from build123d import *

# Parameters (mm, degrees)
SKETCH2_W           = 290
SKETCH2_H           = 165.1
BOSS_EXTRUDE1_DEPTH = 51
SKETCH3_W           = 290
SKETCH3_H           = 165.1
BOSS_EXTRUDE2_DEPTH = 3.175
CUT_EXTRUDE1_DEPTH  = 161.925
SKETCH7_W           = 7.175
SKETCH7_H           = 41.725
CUT_EXTRUDE3_DEPTH  = 158.75
FILLET1_R           = 3.175
SKETCH8_W           = 290
SKETCH8_H           = 6.1
CUT_EXTRUDE4_DEPTH  = 3.25


with BuildPart() as part:
    # Sketch2 → Boss-Extrude1 (new body)
    with BuildSketch(Plane.XY):
        Rectangle(SKETCH2_W, SKETCH2_H)
        Polygon((133.825, 71.375), (133.825, -71.375), (133.825, -79.375), (-133.825, -79.375), (-133.825, -71.375), (-133.825, 71.375), (-133.825, 79.375), (133.825, 79.375), align=None, mode=Mode.SUBTRACT)
    extrude(amount=BOSS_EXTRUDE1_DEPTH)

    # Sketch3 → Boss-Extrude2 (add)
    with BuildSketch(Plane.XY.offset(51)):
        Rectangle(SKETCH3_W, SKETCH3_H)
    extrude(amount=BOSS_EXTRUDE2_DEPTH)

    # Sketch4 → Cut-Extrude1 (cut)
    with BuildSketch(Plane.XZ.offset(82.55)):
        Polygon((140.9, 2.9), (136.9, 2.9), (136.9, 6.1), (145, 6.1), (145, 2.9), (145, 0), (140.9, 0), align=None)
    cut_extrude1 = extrude(amount=-CUT_EXTRUDE1_DEPTH, mode=Mode.SUBTRACT)

    # Mirror1: Cut-Extrude1 across plane
    add(cut_extrude1.mirror(Plane(origin=(0, 0, 0), x_dir=(0, 0, 1), z_dir=(1, 0, 0))), mode=Mode.SUBTRACT)

    # Sketch7 → Cut-Extrude3 (cut)
    with BuildSketch(Plane(origin=(0, 79.375, 0), x_dir=(1, 0, 0), z_dir=(0, 1, 0))):
        with Locations((137.4125, -30.1375)):
            Rectangle(SKETCH7_W, SKETCH7_H)
    cut_extrude3 = extrude(amount=-CUT_EXTRUDE3_DEPTH, mode=Mode.SUBTRACT)

    # Mirror4: Cut-Extrude3 across plane
    add(cut_extrude3.mirror(Plane(origin=(0, 0, 0), x_dir=(0, 0, 1), z_dir=(1, 0, 0))), mode=Mode.SUBTRACT)

    # Fillet1
    fillet1_edges = [part.edges().sort_by_distance(p)[0] for p in [
        (145, -82.55, 30.1375),
        (-145, -82.55, 30.1375),
        (-145, 82.55, 27.0875),
        (145, 82.55, 27.0875),
    ]]
    fillet(fillet1_edges, radius=FILLET1_R)

    # Sketch8 → Cut-Extrude4 (cut)
    with BuildSketch(Plane.XZ.offset(82.55)):
        with Locations((0, 3.05)):
            Rectangle(SKETCH8_W, SKETCH8_H)
    extrude(amount=-CUT_EXTRUDE4_DEPTH, mode=Mode.SUBTRACT)


solid = part.part
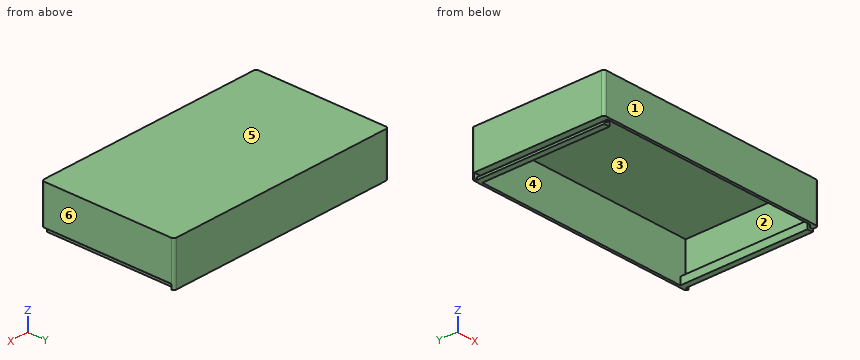
Part model, mm, in its own coordinate system. Face numbers are marked on the shaded views. A direction names the side the tool comes from. Coordinates: 2 decimals unless noted, no trailing zeros. Loops run counter-clockwise (first coordinate to the right, second up) from the corner with the lowest first, then second, coordinate; pieces in that order, holes last. Notation, with made-up numbers: M -23.75,-40 L 34.25,-40 A23 ccw 34.25,-4 Z; hole C -26,59.5 d1. An arc over 180 degrees is marked long. Use a Markdown table: item, result. Add a question column.
Q1. Cut at B-B (z = 13). Write the cut outline in (x, y) (3 decimals).
Q2. Which spindle directions (+Z, -Z, +X, -X, +Y, -Y) get a long thin tool onto all of the face, cutting with end or side? Do the marked faces 1 and 2. Say none if no direction does.
Q3. Probe L1, parallel to X at y = -43.5, z = 16; L2, parallel to Y at x = -6, z = 34 (3 decimals); L3, parallel to X at y = 46, z = 5 (3 decimals). List the from-to ranges inside material, lowest first.
Q4. Cut at C-C (y = 66). Write the cut outline in (x, z) (3 decimals), and give its area (3 significant figures).
Q5. Cut at A-A (x = -12). Write the cut outline in (y, z) (3 decimals).
Q6. Pin check, flat tips, straight feed: P1, Ø2, axis at x = -37, y = 5.5, coming from the -Z side; P2, Ø1.4, axis at y = 29, z = 1, coming from the +X side; P3, Ø5, axis at x = 135.5, z = 2.5, coming from the -Y side; P4, Ø5, axis at x = -139, z = 4.5, coming from the -Y side. Stop position of each tip, or through.
Q7. Mould opens along X. For the marked faces 3, 4, 5 and 6 say: +X half, -X half, draft (parallel to the pull), parting line (faces both ways), or undercut.
Worked out:
| question | item | result |
|---|---|---|
| 1 | outline | M -145,-79.375 A3.175 ccw -141.825,-82.55 L 141.825,-82.55 A3.175 ccw 145,-79.375 L 145,79.375 A3.175 ccw 141.825,82.55 L -141.825,82.55 A3.175 ccw -145,79.375 Z; hole M -141,-79.375 L 141,-79.375 L 141,79.375 L -141,79.375 Z |
| 2 | face 1 | +Z, -Z, +X, -X, -Y |
| 2 | face 2 | none |
| 3 | L1 | x = -145 to -141, 141 to 145 |
| 3 | L2 | y = -82.55 to -79.375, 79.375 to 82.55 |
| 3 | L3 | x = -136.9 to -133.825, 133.825 to 136.9 |
| 4 | outline | M -145,6.1 L -136.9,6.1 L -136.9,2.9 L -140.9,2.9 L -140.9,0 L -133.825,0 L -133.825,9.275 L -141,9.275 L -141,51 L 141,51 L 141,9.275 L 133.825,9.275 L 133.825,0 L 140.9,0 L 140.9,2.9 L 136.9,2.9 L 136.9,6.1 L 145,6.1 L 145,54.175 L -145,54.175 Z |
| 4 | area | 1,390 mm2 |
| 5 | outline | M -82.55,6.1 L -79.375,6.1 L -79.375,51 L 79.375,51 L 79.375,0 L 82.55,0 L 82.55,54.175 L -82.55,54.175 Z |
| 6 | P1 | stops at z = 51 |
| 6 | P2 | stops at x = 140.9 |
| 6 | P3 | stops at y = -79.3 |
| 6 | P4 | stops at y = -82.55 |
| 7 | face 3 | undercut |
| 7 | face 4 | undercut |
| 7 | face 5 | draft |
| 7 | face 6 | +X half |
